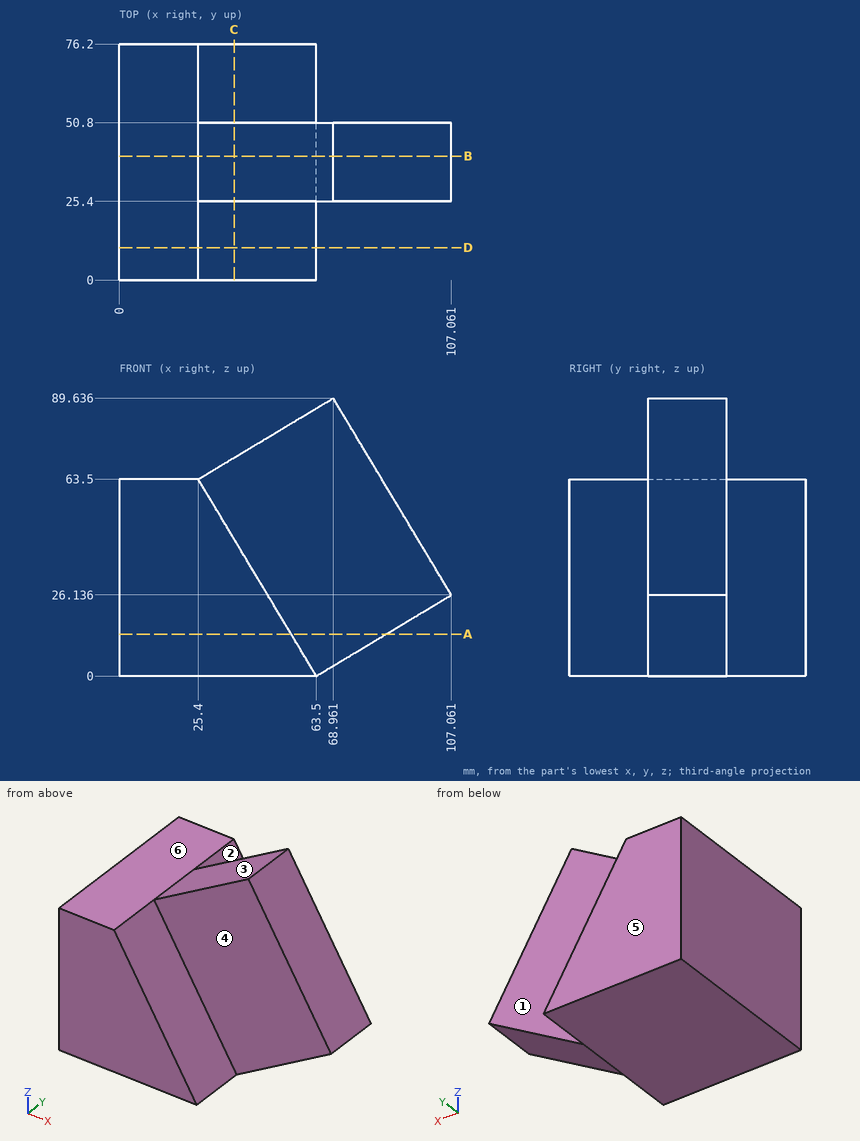
Verification items for this drawing (mm, ordinates from the low corner). A direction names the side the tool comes from. Coordinates: 2 decimals unless noted, no trailing zeros. Loops run counter-clockwise (first coordinate to the right, second up) from the corner with the lowest first, then second, coordinate; pieces in that order, holes last. Notation, with made-up numbers: (19.5, 3) -> (70.5, 3) arc R27 ccw to (70.5, 22) -> close; hole circle Ø1 at (43.5, -6). An arc over 180 degrees is marked (long way). Answer in a Markdown table with one row per item. Add a question column.
1. Material ranges on probe 1 along Y at (x, z) = (86, 21); probe 2 along X at (y, z) = (14, 34.5); probe 3 along Z at (x, y) = (93, 37), recorded low to high. Write a range as [from, to].
2. Section check C-C, the plane x = 37. Enter the section's corners in (y, z), then the cut area to 3 significant figures.
3. Depth check by flat-ended pin: P1, Ø8, axis at x = 40.5, y = 17.5, coming from the +Z side; P2, Ø5, axis at x = 70, y = 55, coming from the -Z side; P3, Ø1, axis at y = 67.5, z = 18, coming from the +X side; P4, Ø7.5, axis at x = 17, y = 31, coming from the +Z side. Enter the tip coordinate at first touch or a pass-through.
4. Access from +Z, -Z, +X, -X, +Y, -Y to the whole of each face (thin tool, end or side, straight path). Record for the marked faces 4, 5 and 6.
5. Section check D-D, the plane y = 10.5. Enter the section's corners in (x, z), then the cut area to 3 significant figures.
6. Section check B-B, the plane y = 40. Enter the section's corners in (x, z).
7. Draft check along X on the marked faces 1, 2 and 3. Enter one of: +X half, -X half, draft (parallel to the pull), parting line (faces both ways), or undercut.
8. Section check A-A, the plane z = 13.5. Enter the section's corners in (x, y), then the cut area to 3 significant figures.
Derived:
| question | item | result |
|---|---|---|
| 1 | probe 1 | y = [25.4, 50.8] |
| 1 | probe 2 | x = [0, 42.8] |
| 1 | probe 3 | z = [17.7, 49.57] |
| 2 | outline | (0, 0) -> (76.2, 0) -> (76.2, 44.17) -> (50.8, 44.17) -> (50.8, 70.46) -> (25.4, 70.46) -> (25.4, 44.17) -> (0, 44.17) -> close |
| 2 | area | 4,030 mm² |
| 3 | P1 | stops at z = 45 |
| 3 | P2 | passes through |
| 3 | P3 | stops at x = 53 |
| 3 | P4 | stops at z = 63.5 |
| 4 | face 4 | +Z, +X, -Y |
| 4 | face 5 | +Z, -Z, +X, -X, +Y |
| 4 | face 6 | +Z, -X, +Y, -Y |
| 5 | outline | (0, 0) -> (63.5, 0) -> (25.4, 63.5) -> (0, 63.5) -> close |
| 5 | area | 2,820 mm² |
| 6 | outline | (0, 0) -> (63.5, 0) -> (107.06, 26.14) -> (68.96, 89.64) -> (25.4, 63.5) -> (0, 63.5) -> close |
| 7 | face 1 | draft |
| 7 | face 2 | +X half |
| 7 | face 3 | -X half |
| 8 | outline | (0, 0) -> (55.4, 0) -> (55.4, 25.4) -> (86, 25.4) -> (86, 50.8) -> (55.4, 50.8) -> (55.4, 76.2) -> (0, 76.2) -> close |
| 8 | area | 5,000 mm² |
